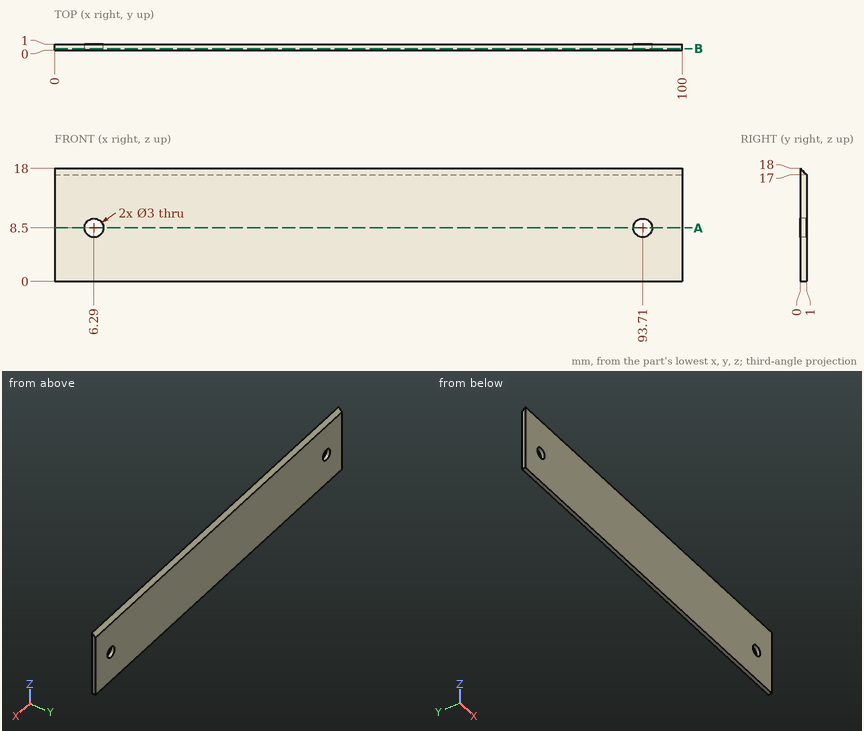
Geometry check sheet. Reference: drawing and pictorial views, mm from the part's lowest x, y, z. Give positions to 0.01 mm unless a question says otherwise; leave off trailing zeros. Order: outer loops, then holes, each group sorted by start corner. A loop starts at its lowest first (then second) coordinate and runs counter-clockwise, first axis right, second up. Notation, with made-up numbers: (47, -25.75) - (61, -25.75) arc R7 cw to (61, -12.75) - close; hole circle Ø7 at (85.5, -1.5). An arc over 180 degrees is marked (long way). Answer as CSV lines item,"result". Start each with the question number.
Item 1: Section check B-B, the plane y = 0.25. Record the boundary of the cut face in (x, z), plus the area to 3 significant figures.
Item 2: Material ranges on L1, parallel to X at y = 0.7, z = 8.5; L2, parallel to X at y = 0.6, z = 9 (1 decimal); L3, parallel to Z at x = 6, y = 0.7, recorded low to high.
Item 3: Section check A-A, the plane z = 8.5. Record the boundary of the cut face in (x, y).
Item 4: Gauge pin test, flat end, axial feed: pin 1 (1.5 mm diameter, centred on x = 86, z = 10, fed in from -Y). Record the tip position at first contact, or that the pin passes through.
Filled in:
1,outline,"(0, 0) - (100, 0) - (100, 17.75) - (0, 17.75) - close; hole circle Ø3 at (6.29, 8.5); hole circle Ø3 at (93.71, 8.5)"
1,area,"1,760 mm^2"
2,L1,"0 to 4.79, 7.79 to 92.21, 95.21 to 100"
2,L2,"0 to 4.9, 7.7 to 92.3, 95.1 to 100"
2,L3,"0 to 7.03, 9.97 to 17.3"
3,outline,"(0, 0) - (4.79, 0) - (4.79, 1) - (0, 1) - close; (7.79, 0) - (92.21, 0) - (92.21, 1) - (7.79, 1) - close; (95.21, 0) - (100, 0) - (100, 1) - (95.21, 1) - close"
4,pin 1,"y = 0"
